Design review of the part built by this model. Coordinates are the model's own, in mm. Face numbers are marked on the shaded views. A direction names the side the tool comes from. Coordinates: 2 decimals unless noted, no trailing zeros. Write each loop counter-clockwise with the first axis right and the second up, starting at its lowest first coordinate (ties: lowest second). Pieces come first, ordered by that corner, then holes.
Autodesk Inventor part; units mm, degrees
ref_plane "Work Plane1" through (0, 0, 4) normal (0, 0, 1) x (1, 0, 0)
ref_plane "YZ Plane" through (0, 0, 0) normal (1, 0, 0) x (0, 1, 0)
ref_plane "XZ Plane" through (0, 0, 0) normal (0, 1, 0) x (-1, 0, 0)
sketch "Sketch1" plane through (0, 0, 0) normal (0, 1, 0) x (-1, 0, 0)
  circle A0 centre (0, 0) radius 2.625
  circle A1 centre (0, 0) radius 4
  dimension "d0" = 5.25
  dimension "d1" = 8
extrude "Extrusion1" add sketch "Sketch1" along normal blind 10
ref_plane "Work Plane1" through (0, 0, 4) normal (0, 0, 1) x (1, 0, 0)
sketch "Sketch2" plane through (0, 0, 4) normal (0, 0, 1) x (1, 0, 0)
  line L0 (4, 10) -> (-4, 10) construction
  line L1 (0, 10) -> (0, 0) construction
  line L2 (0, 10) -> (32, 10)
  line L3 (0, 0) -> (32, 0)
  line L4 (4, 0) -> (-4, 0)
  line L5 (0, 10) -> (0, 0)
  line L6 (32, 0) -> (32, 10)
  dimension "d5" = 32
  dimension "d6" = 32
extrude "Extrusion2" add sketch "Sketch2" against normal blind 1.375
sketch "Sketch3" plane through (0, 0, 4) normal (0, 0, 1) x (1, 0, 0)
  line L0 (-2.625, 10) -> (2.625, 10)
  line L1 (0, 10) -> (0, 0)
  line L2 (0, 0) -> (6, 0)
  line L3 (32, 0) -> (3.0182, 0)
  line L4 (6, 0) -> (6, 10)
  line L5 (6, 10) -> (0, 10)
  dimension "d9" = 6
extrude "Extrusion3" add sketch "Sketch3" along normal blind 6
sketch "Sketch4" plane through (0, 0, 4) normal (-1, 0, 0) x (0, 0, 1)
  line L0 (6, 0) -> (6, 10) construction
  line L1 (6, 5) -> (0, 5) construction
  line L2 (0, 0) -> (0, 10) construction
  line L3 (0, 5) -> (0, 8.125)
  line L4 (0, 5) -> (0, 1.875)
  line L5 (0, 1.875) -> (4.25, 1.875)
  line L6 (4.25, 1.875) -> (4.25, 8.125)
  line L7 (4.25, 8.125) -> (0, 8.125)
  point P0 (-4, 0)
  dimension "d12" = 3.125
  dimension "d13" = 3.125
  dimension "d14" = 4.25
extrude "Extrusion4" cut sketch "Sketch4" against normal up to next
sketch "Sketch5" plane through (0, 0, 4) normal (0, 0, 1) x (1, 0, 0)
  line L0 (32, 10) -> (28, 10)
  line L1 (32, 10) -> (6, 10)
  line L2 (28, 10) -> (28, 0)
  line L3 (6, 0) -> (32, 0)
  line L4 (32, 0) -> (28, 0)
  line L5 (32, 0) -> (32, 10)
  point P0 (0, 0)
  dimension "d17" = 4
extrude "Extrusion5" add sketch "Sketch5" along normal blind 3
sketch "Sketch6" plane through (28, 0, 4) normal (-1, 0, 0) x (0, 0, 1)
  line L0 (-1.375, 10) -> (3, 10) construction
  line L1 (3, 10) -> (3, 0) construction
  line L2 (0, 0) -> (6, 0) construction
  line L3 (3, 0) -> (3, 10) construction
  line L4 (3, 5) -> (0, 5) construction
  line L5 (0, 1.875) -> (0, 8.125) construction
  line L6 (0, 5) -> (0, 6.625)
  line L7 (0, 5) -> (0, 3.375)
  line L8 (0, 3.375) -> (2, 3.375)
  line L9 (2, 3.375) -> (2, 6.625)
  line L10 (2, 6.625) -> (0, 6.625)
  point P0 (-4, 0)
  dimension "d20" = 1.625
  dimension "d21" = 1.625
  dimension "d22" = 2
extrude "Extrusion6" cut sketch "Sketch6" against normal up to next
properties part number "tiny LED's standoff mount"
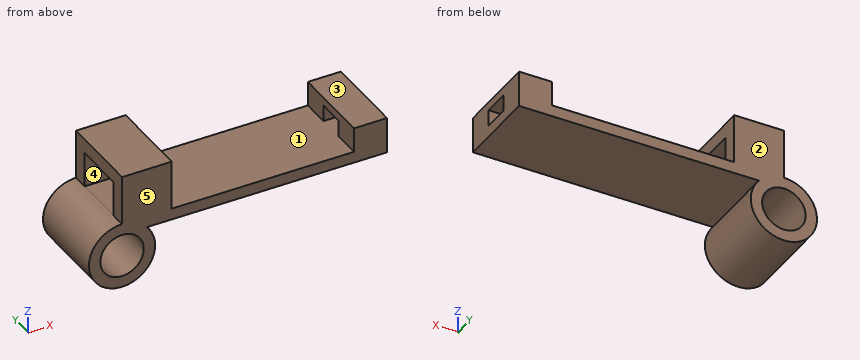
(1) Consider section B-B (z = 0). Give the boundary of the cut face in (x, y) (3 decimals), plus the area to 3 significant figures.
(2) Consider section C-C (x = 28.5). Give the boundary of the cut face in (y, z) (3 decimals).
(3) Insertion check: pin 1 Ø1.8 at (x, y) = (2, 6) entering from -Z; pin 2 Ø5 at (x, y) = (25, 7.5) entering from -Z (3 decimals); pin 3 Ø2 at (y, z) = (5.5, -2) entering from +X. Each pin has a flat end and moves straight along its axis. Give the tip position at first contact, or say it passes through.
(4) Consider section D-D (x = -1). Give the boundary of the cut face in (y, z).
(5) Wall thickness on line 1 (X direction, y = 4, z = 0) (3 decimals); line 2 (X direction, y = 2, z = 4.5); line 3 (Z direction, x = 29.5, y = 6.75) (3 decimals): over which ranges is each line inside the solid? List them lowest first.
(6) For the marked faces 4 and 5, list the 3-axis set-ups (+Z, -Z, +X, -X, +Y, -Y) from which the entire face can be reached by the end or side of a thin tool; tool diameter is ignored.
(7) Consider section A-A (y = 4.5). Give the boundary of the cut face in (x, z) (3 decimals), plus the area to 3 significant figures.
(8) Mouldability with a two-part tool opening along Y and no side actions: class the marked faces 1, 2 and 3 as +Y half, -Y half, draft (parallel to the pull), parting line (faces both ways), or undercut.
Results:
1. outline: (-4, 0) - (-2.625, 0) - (-2.625, 10) - (-4, 10) - close; (2.625, 0) - (4, 0) - (4, 10) - (2.625, 10) - close
1. area: 27.5 mm2
2. outline: (0, 2.625) - (10, 2.625) - (10, 7) - (0, 7) - close; hole (3.375, 4) - (6.625, 4) - (6.625, 6) - (3.375, 6) - close
3. pin 1: stops at z = -3.85
3. pin 2: stops at z = 2.625
3. pin 3: stops at x = 3.87
4. outline: (0, -3.87) - (10, -3.87) - (10, -2.43) - (0, -2.43) - close; (0, 2.43) - (10, 2.43) - (10, 3.87) - (0, 3.87) - close
5. line 1: x = -4 to -2.625, 2.625 to 4
5. line 2: x = 28 to 32
5. line 3: z = 2.625 to 7
6. face 4: -X
6. face 5: +Z, -Z, +X, -X, -Y
7. outline: (0, 4) arc R4 ccw (long way) to (3.018, 2.625) - (32, 2.625) - (32, 4) - close; (0, 8.25) - (6, 8.25) - (6, 10) - (0, 10) - close; (28, 6) - (32, 6) - (32, 7) - (28, 7) - close; hole circle Ø5.25 at (0, 0)
7. area: 84.2 mm2
8. face 1: undercut
8. face 2: +Y half
8. face 3: draft
